For this review, take the finished solid that the model builds, in its own axes (mm). A direction names the side the tool comes from. Give positions to 0.01 mm unless a question says otherwise; leave off trailing zeros. Order: outer loops, then holes, each group sorted by start corner. A loop starts at its lowest first (then second) coordinate and runs counter-clockwise, first axis right, second up.
from build123d import *

# Parameters (mm, degrees)
SKETCH1_R           = 2.5
BOSS_EXTRUDE1_DEPTH = 15
SKETCH2_R           = 4.95
BOSS_EXTRUDE2_DEPTH = 5.5
SKETCH7_W           = 1.8
SKETCH7_H           = 5.6
CUT_EXTRUDE3_DEPTH  = 5.5
SKETCH10_R          = 2.5
CUT_EXTRUDE4_DEPTH  = 23.053457779
SKETCH13_W          = 1.7
SKETCH13_H          = 2.55
BOSS_EXTRUDE5_START = 1
SKETCH14_R          = 6
BOSS_EXTRUDE5_DEPTH = 1


with BuildPart() as part:
    # Sketch1 → Boss-Extrude1 (new body)
    with BuildSketch(Plane(origin=(0, 0, 0), x_dir=(1, 0, 0), z_dir=(0, 1, 0))):
        with Locations(Location((0, 0, 0), (0, 0, 270))):
            Circle(SKETCH1_R)
    extrude(amount=BOSS_EXTRUDE1_DEPTH)

    # Sketch2 → Boss-Extrude2 (add)
    with BuildSketch(Plane(origin=(0, 15, 0), x_dir=(1, 0, 0), z_dir=(0, 1, 0))):
        with Locations(Location((1.5, 0, 0), (0, 0, 270))):
            Circle(SKETCH2_R)
    extrude(amount=BOSS_EXTRUDE2_DEPTH)

    # Sketch7 → Cut-Extrude3 (cut)
    with BuildSketch(Plane.XZ.offset(-15)):
        with Locations((3, 0)):
            Rectangle(SKETCH7_W, SKETCH7_H)
    extrude(amount=-CUT_EXTRUDE3_DEPTH, mode=Mode.SUBTRACT)

    # Sketch10 → Cut-Extrude4 (cut, through all)
    with BuildSketch(Plane.XZ):
        Circle(SKETCH10_R)
    extrude(amount=-CUT_EXTRUDE4_DEPTH, mode=Mode.SUBTRACT)

    # Sketch13 → M3 Clearance Hole1 (revolve, cut)
    with BuildSketch(Plane(origin=(3.9, 17.75, 0), x_dir=(0, 0, 1), z_dir=(0, 1, 0))):
        with Locations((0.85, 1.275)):
            Rectangle(SKETCH13_W, SKETCH13_H)
    revolve(axis=Axis((-2.45, 17.75, 0), (1, 0, 0)), mode=Mode.SUBTRACT)

    # Sketch14 → Boss-Extrude5 (add)
    with BuildSketch(Plane.XZ.offset(-15).offset(BOSS_EXTRUDE5_START)):
        with Locations(Location((1.5, 0, 0), (0, 0, 270))):
            Circle(SKETCH14_R)
        with BuildLine():
            Line((2.1, 2.8), (2.1, 1.356465997))
            ThreePointArc((2.1, 1.356465997), (-2.5, 0), (2.1, -1.356465997))
            Line((2.1, -1.356465997), (2.1, -2.8))
            Line((2.1, -2.8), (3.9, -2.8))
            Line((3.9, -2.8), (3.9, 2.8))
            Line((3.9, 2.8), (2.1, 2.8))
        make_face(mode=Mode.SUBTRACT)
    extrude(amount=-BOSS_EXTRUDE5_DEPTH)


solid = part.part
1) Draft analysis for pull direction X (two halves, no side actions). For faces 1 (the face through (-0.8, 14.49, -5.54)), 2 (the face through (6.42, 15, 1.36)), 3 (the face through (3, 17, -2.8)), state which applies: +X half, -X half, draft (parallel to the pull), parting line (faces both ways), or undercut.
Answer sheet:
face 1: parting line
face 2: draft
face 3: undercut
2) We need section D-D on y = 18.75. Give the boundary of the cut face in (x, z).
Answer sheet:
outline: (2.1, -2.8) - (2.1, -1.36) arc R2.5 cw (long way) to (2.1, 1.36) - (2.1, 2.8) - (3.9, 2.8) - (3.9, 1.37) - (6.26, 1.37) arc R4.95 ccw (long way) to (6.26, -1.37) - (3.9, -1.37) - (3.9, -2.8) - close
3) To check wall thickness, follow line 1 (X direction, y = 18, z = 2.25); line 2 (Y direction, x = -3, z = -2.5); line 3 (X direction, y = 14.45, z = 0). State the ranges of each line that lie inside material, in increasing order.
Answer sheet:
line 1: x = -2.91 to -1.09, 1.09 to 2.1, 3.9 to 5.91
line 2: y = 14 to 15
line 3: x = -4.5 to -2.5, 3.9 to 7.5
4) Clearance check with flat-ended pins moving along their axes: pin 1 (0.9 mm diameter, centred on x = 2.5, y = 16.5, fed in from +Z); pin 2 (0.7 mm diameter, centred on y = 16.5, z = 2, fed in from +X); pin 3 (2 mm diameter, centred on x = 3.5, y = 16.5, fed in from -Z). State where each tip first meets the part, or that it passes through.
Answer sheet:
pin 1: stops at z = 4.92
pin 2: stops at x = 6.17
pin 3: stops at z = -4.85
5) We need section B-B on x = 1.5. Give the boundary of the cut face in (y, z).
Answer sheet:
outline: (14, -6) - (15, -6) - (15, -4.95) - (20.5, -4.95) - (20.5, -2) - (14, -2) - close; (14, 2) - (20.5, 2) - (20.5, 4.95) - (15, 4.95) - (15, 6) - (14, 6) - close
6) We need section A-A on z = 0. Give the boundary of the cut face in (x, y).
Answer sheet:
outline: (-4.5, 14) - (-2.5, 14) - (-2.5, 20.5) - (-3.45, 20.5) - (-3.45, 15) - (-4.5, 15) - close; (3.9, 14) - (7.5, 14) - (7.5, 15) - (6.45, 15) - (6.45, 16.05) - (3.9, 16.05) - close; (3.9, 19.45) - (6.45, 19.45) - (6.45, 20.5) - (3.9, 20.5) - close
7) Tool access review of faces 4 (the face through (5.19, 18.4, 1.57)), 5 (the face through (-3.332, 17.712, -1.073)), 6 (the face through (2.1, 17, -2)): name each direction out of +Z, -Z, +X, -X, +Y, -Y from which nothing blocks a thin tool from reaching the whole face with its end or side.
Answer sheet:
face 4: +X
face 5: +Y
face 6: +Y, -Y
8) We need section C-C on x = 5.75. Give the boundary of the cut face in (y, z).
Answer sheet:
outline: (14, -4.24) - (15, -4.24) - (15, -2.54) - (20.5, -2.54) - (20.5, 2.54) - (15, 2.54) - (15, 4.24) - (14, 4.24) - close; hole circle Ø3.4 at (17.75, 0)
